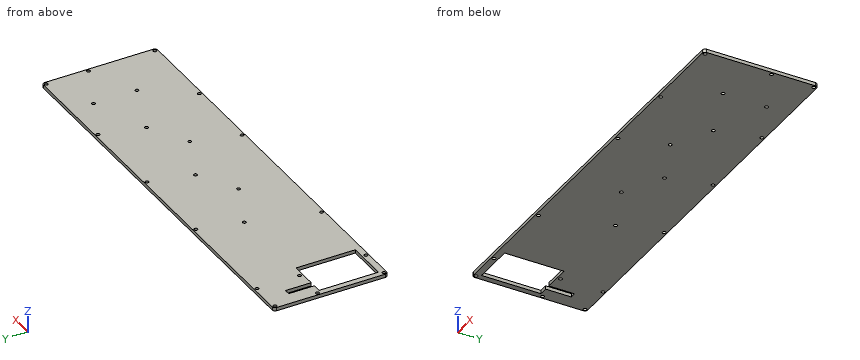
Autodesk Fusion 360 part; units mm, degrees
sketch "Sketch1" plane through (0, 0, 0) normal (0, 0, 1) x (1, 0, 0)
  circle A0 centre (317.6723, -113.9909) radius 1.5
  circle A1 centre (386.7293, -18.6469) radius 1.5
  line L0 (30.0243, -116.3719) -> (386.7293, -116.3719)
  circle A2 centre (229.5683, -18.5529) radius 1.5
  circle A3 centre (262.9063, -74.7719) radius 1.5
  line L1 (389.2043, -113.8969) -> (389.2043, -18.6469)
  arc A4 (389.2043, -18.6469) -> (386.7293, -16.1719) centre (386.7293, -18.6469) ccw
  circle A5 centre (143.8433, -55.7219) radius 1.5
  circle A6 centre (296.2433, -55.7219) radius 1.5
  line L2 (386.7293, -16.1719) -> (30.0243, -16.1719)
  circle A7 centre (305.7683, -18.5529) radius 1.5
  circle A8 centre (386.7293, -55.7219) radius 1.5
  circle A9 centre (153.3663, -18.5529) radius 1.5
  arc A10 (27.6433, -113.9909) -> (30.0243, -116.3719) centre (30.0243, -113.9909) ccw
  circle A11 centre (58.0243, -55.7219) radius 1.5
  circle A12 centre (30.0243, -18.5529) radius 1.5
  circle A13 centre (250.9983, -113.9909) radius 1.5
  line L3 (27.6433, -18.5529) -> (27.6433, -113.9909)
  circle A14 centre (58.0243, -18.5529) radius 1.5
  arc A15 (30.0243, -16.1719) -> (27.6433, -18.5529) centre (30.0243, -18.5529) ccw
  circle A16 centre (127.1733, -113.9909) radius 1.5
  arc A17 (386.7293, -116.3719) -> (389.2043, -113.8969) centre (386.7293, -113.8969) ccw
  circle A18 centre (386.7293, -113.8969) radius 1.5
  circle A19 centre (30.0243, -55.7219) radius 1.5
  circle A20 centre (345.1433, -74.7719) radius 1.5
  circle A21 centre (30.0243, -113.9909) radius 1.5
  circle A22 centre (220.0433, -55.7219) radius 1.5
  circle A23 centre (58.0243, -113.9909) radius 1.5
  circle A24 centre (186.7063, -74.7719) radius 1.5
  circle A25 centre (345.1433, -36.6719) radius 1.5
  point P0 (389.2043, -16.1719)
  point P1 (27.6433, -16.1719)
  point P2 (389.2043, -116.3719)
  dimension "d78" = 100.2
  dimension "d79" = 361.561
  dimension "d80" = 3
  dimension "d81" = 2.381
  dimension "d82" = 2.381
  dimension "d83" = 30.381
  dimension "d84" = 125.723
  dimension "d85" = 201.925
  dimension "d86" = 278.125
  dimension "d87" = 2.475
  dimension "d88" = 2.475
  dimension "d89" = 2.381
  dimension "d90" = 2.381
  dimension "d91" = 2.381
  dimension "d92" = 2.381
  dimension "d93" = 3
  dimension "d94" = 3
  dimension "d95" = 3
  dimension "d96" = 3
  dimension "d97" = 3
  dimension "d98" = 2.381
  dimension "d99" = 2.381
  dimension "d100" = 2.381
  dimension "d101" = 2.381
  dimension "d102" = 2.381
  dimension "d103" = 2.381
  dimension "d104" = 2.381
  dimension "d105" = 2.475
  dimension "d106" = 2.475
  dimension "d107" = 2.475
  dimension "d108" = 39.55
  dimension "d109" = 39.55
  dimension "d110" = 39.55
  dimension "d111" = 39.55
  dimension "d112" = 39.55
  dimension "d113" = 39.55
  dimension "d114" = 30.381
  dimension "d115" = 116.2
  dimension "d116" = 192.4
  dimension "d117" = 268.6
  dimension "d118" = 44.061
  dimension "d119" = 20.5
  dimension "d120" = 3
  dimension "d121" = 3
  dimension "d122" = 3
  dimension "d123" = 3
  dimension "d124" = 3
  dimension "d125" = 3
  dimension "d126" = 30.381
  dimension "d127" = 99.53
  dimension "d128" = 223.355
  dimension "d129" = 290.029
  dimension "d130" = 44.061
  dimension "d131" = 58.6
  dimension "d132" = 159.063
  dimension "d133" = 235.263
  dimension "d134" = 41.6
  dimension "d135" = 41.6
  dimension "d136" = 3
  dimension "d137" = 3
  dimension "d138" = 3
  dimension "d139" = 3
  dimension "d140" = 3
  dimension "d141" = 3
  dimension "d142" = 3
  dimension "d143" = 3
  dimension "d144" = 3
  dimension "d145" = 3
  dimension "d146" = 2.381
  dimension "d147" = 2.381
  dimension "d148" = 2.475
  dimension "d149" = 2.475
extrude "Extrude1" add sketch "Sketch1" along normal blind 3
sketch "Sketch2" plane through (0, 0, 3) normal (0, 0, 1) x (-1, 0, 0)
  circle A0 centre (-143.8433, 55.7219) radius 1.5
  circle A1 centre (-386.7293, 113.8969) radius 1.5
  circle A2 centre (-262.9063, 74.7719) radius 1.5
  circle A3 centre (-30.0243, 113.9909) radius 1.5
  circle A4 centre (-58.0243, 55.7219) radius 1.5
  circle A5 centre (-250.9983, 113.9909) radius 1.5
  circle A6 centre (-317.6723, 113.9909) radius 1.5
  circle A7 centre (-296.2433, 55.7219) radius 1.5
  circle A8 centre (-127.1733, 113.9909) radius 1.5
  circle A9 centre (-386.7293, 55.7219) radius 1.5
  circle A10 centre (-386.7293, 18.6469) radius 1.5
  circle A11 centre (-345.1433, 74.7719) radius 1.5
  circle A12 centre (-58.0243, 18.5529) radius 1.5
  circle A13 centre (-30.0243, 18.5529) radius 1.5
  circle A14 centre (-186.7063, 74.7719) radius 1.5
  circle A15 centre (-345.1433, 36.6719) radius 1.5
  circle A16 centre (-153.3663, 18.5529) radius 1.5
  circle A17 centre (-305.7683, 18.5529) radius 1.5
  circle A18 centre (-229.5683, 18.5529) radius 1.5
  circle A19 centre (-58.0243, 113.9909) radius 1.5
  circle A20 centre (-30.0243, 55.7219) radius 1.5
  circle A21 centre (-220.0433, 55.7219) radius 1.5
  arc A22 (-386.7293, 116.3719) -> (-389.2043, 113.8969) centre (-386.7293, 113.8969) ccw
  line L0 (-389.2043, 113.8969) -> (-389.2043, 18.6469)
  arc A23 (-389.2043, 18.6469) -> (-386.7293, 16.1719) centre (-386.7293, 18.6469) ccw
  line L1 (-386.7293, 16.1719) -> (-30.0243, 16.1719)
  arc A24 (-30.0243, 16.1719) -> (-27.6433, 18.5529) centre (-30.0243, 18.5529) ccw
  line L2 (-27.6433, 18.5529) -> (-27.6433, 113.9909)
  arc A25 (-27.6433, 113.9909) -> (-30.0243, 116.3719) centre (-30.0243, 113.9909) ccw
  line L3 (-30.0243, 116.3719) -> (-386.7293, 116.3719)
  line L4 (-32.6433, 58.7219) -> (-68.6433, 58.7219)
  line L5 (-68.6433, 58.7219) -> (-68.6433, 110.7219)
  line L6 (-68.6433, 110.7219) -> (-32.6433, 110.7219)
  line L7 (-32.6433, 110.7219) -> (-32.6433, 58.7219)
  line L8 (-40, 36.1719) -> (-45, 36.1719)
  line L9 (-45, 36.1719) -> (-45, 58.7219)
  line L10 (-45, 58.7219) -> (-40, 58.7219)
  line L11 (-40, 58.7219) -> (-40, 36.1719)
  dimension "d153" = 36
  dimension "d154" = 52
  dimension "d155" = 3
  dimension "d156" = 5
  dimension "d159" = 5
  dimension "d161" = 20
extrude "Extrude2" cut sketch "Sketch2" against normal blind 3 contours L4 L5 L6 L7 L10 | L4 L8 L9 L10 L11
sketch "Sketch3" plane through (0, 0, 3) normal (0, 0, 1) x (-1, 0, 0)
  line L0 (-68.6433, 58.7219) -> (-68.6433, 110.7219)
  line L1 (-68.6433, 110.7219) -> (-32.6433, 110.7219)
  line L2 (-32.6433, 110.7219) -> (-32.6433, 58.7219)
  line L3 (-32.6433, 58.7219) -> (-40, 58.7219)
  circle A0 centre (-143.8433, 55.7219) radius 1.5
  circle A1 centre (-386.7293, 113.8969) radius 1.5
  circle A2 centre (-262.9063, 74.7719) radius 1.5
  circle A3 centre (-30.0243, 113.9909) radius 1.5
  circle A4 centre (-58.0243, 55.7219) radius 1.5
  circle A5 centre (-250.9983, 113.9909) radius 1.5
  circle A6 centre (-317.6723, 113.9909) radius 1.5
  circle A7 centre (-296.2433, 55.7219) radius 1.5
  circle A8 centre (-127.1733, 113.9909) radius 1.5
  circle A9 centre (-386.7293, 55.7219) radius 1.5
  circle A10 centre (-386.7293, 18.6469) radius 1.5
  circle A11 centre (-345.1433, 74.7719) radius 1.5
  circle A12 centre (-58.0243, 18.5529) radius 1.5
  circle A13 centre (-30.0243, 18.5529) radius 1.5
  circle A14 centre (-186.7063, 74.7719) radius 1.5
  circle A15 centre (-345.1433, 36.6719) radius 1.5
  circle A16 centre (-153.3663, 18.5529) radius 1.5
  circle A17 centre (-305.7683, 18.5529) radius 1.5
  circle A18 centre (-229.5683, 18.5529) radius 1.5
  circle A19 centre (-58.0243, 113.9909) radius 1.5
  circle A20 centre (-30.0243, 55.7219) radius 1.5
  circle A21 centre (-220.0433, 55.7219) radius 1.5
  arc A22 (-386.7293, 116.3719) -> (-389.2043, 113.8969) centre (-386.7293, 113.8969) ccw
  line L4 (-389.2043, 113.8969) -> (-389.2043, 18.6469)
  arc A23 (-389.2043, 18.6469) -> (-386.7293, 16.1719) centre (-386.7293, 18.6469) ccw
  line L5 (-386.7293, 16.1719) -> (-30.0243, 16.1719)
  arc A24 (-30.0243, 16.1719) -> (-27.6433, 18.5529) centre (-30.0243, 18.5529) ccw
  line L6 (-27.6433, 18.5529) -> (-27.6433, 113.9909)
  arc A25 (-27.6433, 113.9909) -> (-30.0243, 116.3719) centre (-30.0243, 113.9909) ccw
  line L7 (-30.0243, 116.3719) -> (-386.7293, 116.3719)
  line L8 (-40, 58.7219) -> (-40, 36.1719)
  line L9 (-40, 36.1719) -> (-45, 36.1719)
  line L10 (-45, 36.1719) -> (-45, 58.7219)
  line L11 (-45, 58.7219) -> (-68.6433, 58.7219)
sketch "Sketch4" plane through (0, 0, 3) normal (0, 0, 1) x (-1, 0, 0)
  line L0 (-68.6433, 58.7219) -> (-68.6433, 110.7219)
  line L1 (-68.6433, 110.7219) -> (-32.6433, 110.7219)
  line L2 (-32.6433, 110.7219) -> (-32.6433, 58.7219)
  line L3 (-32.6433, 58.7219) -> (-40, 58.7219)
  circle A0 centre (-143.8433, 55.7219) radius 1.5
  circle A1 centre (-386.7293, 113.8969) radius 1.5
  circle A2 centre (-262.9063, 74.7719) radius 1.5
  circle A3 centre (-30.0243, 113.9909) radius 1.5
  circle A4 centre (-58.0243, 55.7219) radius 1.5
  circle A5 centre (-250.9983, 113.9909) radius 1.5
  circle A6 centre (-317.6723, 113.9909) radius 1.5
  circle A7 centre (-296.2433, 55.7219) radius 1.5
  circle A8 centre (-127.1733, 113.9909) radius 1.5
  circle A9 centre (-386.7293, 55.7219) radius 1.5
  circle A10 centre (-386.7293, 18.6469) radius 1.5
  circle A11 centre (-345.1433, 74.7719) radius 1.5
  circle A12 centre (-58.0243, 18.5529) radius 1.5
  circle A13 centre (-30.0243, 18.5529) radius 1.5
  circle A14 centre (-186.7063, 74.7719) radius 1.5
  circle A15 centre (-345.1433, 36.6719) radius 1.5
  circle A16 centre (-153.3663, 18.5529) radius 1.5
  circle A17 centre (-305.7683, 18.5529) radius 1.5
  circle A18 centre (-229.5683, 18.5529) radius 1.5
  circle A19 centre (-58.0243, 113.9909) radius 1.5
  circle A20 centre (-30.0243, 55.7219) radius 1.5
  circle A21 centre (-220.0433, 55.7219) radius 1.5
  arc A22 (-386.7293, 116.3719) -> (-389.2043, 113.8969) centre (-386.7293, 113.8969) ccw
  line L4 (-389.2043, 113.8969) -> (-389.2043, 18.6469)
  arc A23 (-389.2043, 18.6469) -> (-386.7293, 16.1719) centre (-386.7293, 18.6469) ccw
  line L5 (-386.7293, 16.1719) -> (-30.0243, 16.1719)
  arc A24 (-30.0243, 16.1719) -> (-27.6433, 18.5529) centre (-30.0243, 18.5529) ccw
  line L6 (-27.6433, 18.5529) -> (-27.6433, 113.9909)
  arc A25 (-27.6433, 113.9909) -> (-30.0243, 116.3719) centre (-30.0243, 113.9909) ccw
  line L7 (-30.0243, 116.3719) -> (-386.7293, 116.3719)
  line L8 (-40, 58.7219) -> (-40, 36.1719)
  line L9 (-40, 36.1719) -> (-45, 36.1719)
  line L10 (-45, 36.1719) -> (-45, 58.7219)
  line L11 (-45, 58.7219) -> (-68.6433, 58.7219)
equation "d80 = m2_hole_standoff"
equation "d93 = m2_hole_standoff"
equation "d94 = m2_hole_standoff"
equation "d95 = m2_hole_standoff"
equation "d96 = m2_hole_standoff"
equation "d97 = m2_hole_standoff"
equation "d120 = m2_hole_standoff"
equation "d121 = m2_hole_standoff"
equation "d122 = m2_hole_standoff"
equation "d123 = m2_hole_standoff"
equation "d124 = m2_hole_standoff"
equation "d125 = m2_hole_standoff"
equation "d136 = m2_hole_standoff"
equation "d137 = m2_hole_standoff"
equation "d138 = m2_hole_standoff"
equation "d139 = m2_hole_standoff"
equation "d140 = m2_hole_standoff"
equation "d141 = m2_hole_standoff"
equation "d142 = m2_hole_standoff"
equation "d143 = m2_hole_standoff"
equation "d144 = m2_hole_standoff"
equation "d145 = m2_hole_standoff"
equation "m2_hole_standoff = 3 mm"
Geometry: final body of the model. Coordinates: model frame, mm. Round coordinates to 2 decimals unless told otherwise and drop trailing zeros. Loops run counter-clockwise (first coordinate to the right, second up) from the corner with the lowest first, then second, coordinate; pieces in that order, holes last. Notation, with made-up numbers: M -16.5,-24.5 L 12.5,-24.5 A17 ccw 12.5,-6.5 Z; hole C 75,51.25 d3. An arc over 180 degrees is marked long. One line per question, with ' | ' between items.
(1) Material intervals for line 1 along Y through (x, z) = (54, 2.35); line 2 along X through (y, z) = (-70.5, 0.65); line 3 along X through (y, z) = (-39, 1.2), sorted ascending. Write a range as from..to.
Check result:
line 1: y = -116.37..-110.72, -58.72..-16.17 | line 2: x = 27.64..32.64, 68.64..389.2 | line 3: x = 27.64..40, 45..389.2
(2) Cut plane A-A on x = 52.5. Return the cut outline in (y, z), plus the area to 3 significant figures.
Check result:
outline: M -116.37,0 L -110.72,0 L -110.72,3 L -116.37,3 Z; M -58.72,0 L -16.17,0 L -16.17,3 L -58.72,3 Z | area: 145 mm2
(3) Cut plane B-B on y = -67. Return the cut outline in (x, z), plus the area to 3 significant figures.
Check result:
outline: M 27.64,0 L 32.64,0 L 32.64,3 L 27.64,3 Z; M 68.64,0 L 389.2,0 L 389.2,3 L 68.64,3 Z | area: 977 mm2
(4) Cut plane C-C on z = 0.45. Give the number of separate pieces and of enclosed holes in the cut face, plus the area to 3 significant figures.
Check result:
separate pieces: 1 | enclosed holes: 23 | area: 34,100 mm2
